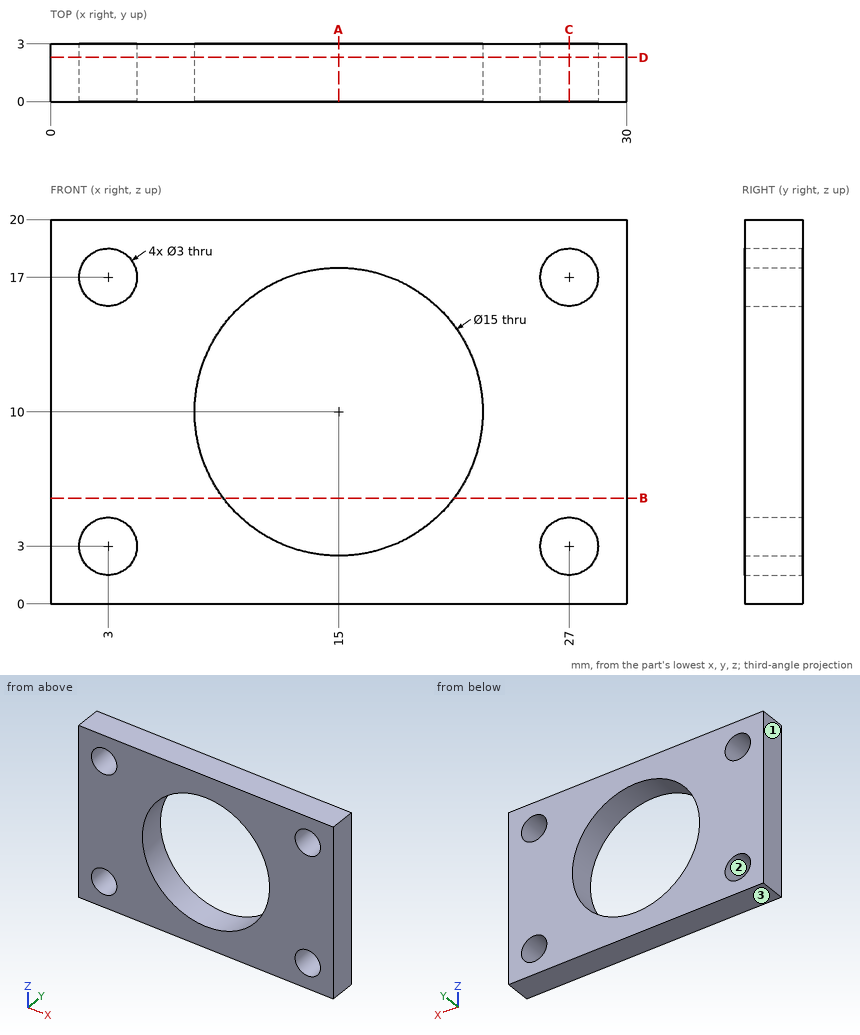
Answer from the drawing. Dimensions are ordinates in mm from the lowest x, y and z of the part. Coordinates: 2 decimals unless noted, no trailing zeros. Write each loop counter-clockwise with the first axis right and the second up, starting at its lowest first coordinate (ties: lowest second). Pieces come first, ordered by that corner, then holes. Notation, with made-up numbers: (75, 4.5) -> (94, 4.5) arc R7 ccw to (94, 9.5) -> close; hole circle Ø7 at (-1, 83). An arc over 180 degrees is marked (long way). One line per question, with ' | ' between items.
1. Section C-C (x = 27) is taken. Determine the outline of the cut face in (y, z), and give its area (3 significant figures).
Verdict:
outline: (0, 0) -> (3, 0) -> (3, 1.5) -> (0, 1.5) -> close; (0, 4.5) -> (3, 4.5) -> (3, 15.5) -> (0, 15.5) -> close; (0, 18.5) -> (3, 18.5) -> (3, 20) -> (0, 20) -> close | area: 42.0 mm^2
2. Section B-B (z = 5.5) is taken. Determine the outline of the cut face in (x, y), and give its area (3 significant figures).
Verdict:
outline: (0, 0) -> (9, 0) -> (9, 3) -> (0, 3) -> close; (21, 0) -> (30, 0) -> (30, 3) -> (21, 3) -> close | area: 54.0 mm^2
3. For a pull along Z with two mould halves and no side action, classify the marked faces 1, 2 and 3 as released by +Z, released by -Z, zero draft, split by the parting line, or undercut.
Verdict:
face 1: zero draft | face 2: undercut | face 3: released by -Z
4. Section A-A (x = 15) is taken. Determine the outline of the cut face in (y, z), and give its area (3 significant figures).
Verdict:
outline: (0, 0) -> (3, 0) -> (3, 2.5) -> (0, 2.5) -> close; (0, 17.5) -> (3, 17.5) -> (3, 20) -> (0, 20) -> close | area: 15.0 mm^2
5. Straight lines are drawn through the part: line 1 (Z direction, x = 3, y = 1.95); line 2 (X direction, y = 1.95, z = 10); line 3 (Z direction, x = 15, y = 1.45). For each, find the intervals that lie inside material, in ascending order.
Verdict:
line 1: z = 0 to 1.5, 4.5 to 15.5, 18.5 to 20 | line 2: x = 0 to 7.5, 22.5 to 30 | line 3: z = 0 to 2.5, 17.5 to 20
6. Given pin 1 Ø2.5 at (x, z) = (27, 3) entering from +Y, flat-ended and moving along its own axis, determine where the tip first touches the part or whether it passes through.
Verdict:
pin 1: passes through
7. Section D-D (y = 2.3) is taken. Determine the outline of the cut face in (x, z), and give its area (3 significant figures).
Verdict:
outline: (0, 0) -> (30, 0) -> (30, 20) -> (0, 20) -> close; hole circle Ø3 at (3, 3); hole circle Ø3 at (3, 17); hole circle Ø15 at (15, 10); hole circle Ø3 at (27, 3); hole circle Ø3 at (27, 17) | area: 395 mm^2
